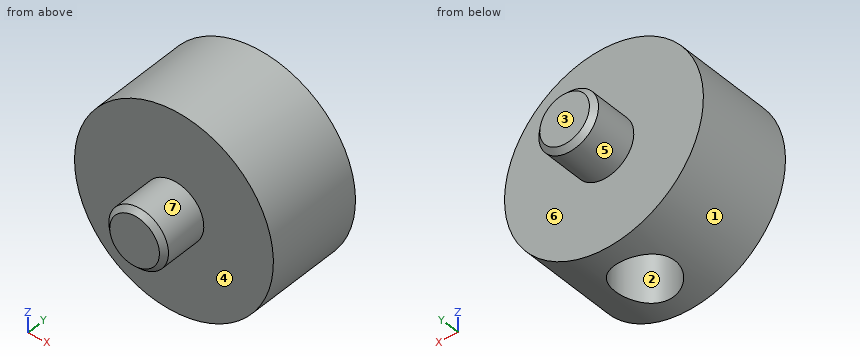
from build123d import *

# Parameters (mm, degrees)
SCHIZZO1_R                   = 10
ESTRUSIONE_ESTRUSIONE1_DEPTH = 10
ESTRUSIONE_ESTRUSIONE2_START = -14.8
SCHIZZO2_R                   = 3
ESTRUSIONE_ESTRUSIONE2_DEPTH = 19.6
TAGLIO_ESTRUSIONE1_START     = -0.5
SCHIZZO3_R                   = 3
TAGLIO_ESTRUSIONE1_DEPTH     = 9.5
SMUSSO1_SIZE                 = 0.5


with BuildPart() as part:
    # Schizzo1 → Estrusione-Estrusione1 (new body)
    with BuildSketch(Plane(origin=(0, 0, 0), x_dir=(1, 0, 0), z_dir=(0, 1, 0))):
        with Locations(Location((0, 0, 0), (0, 0, 270))):
            Circle(SCHIZZO1_R)
    extrude(amount=ESTRUSIONE_ESTRUSIONE1_DEPTH)

    # Schizzo2 → Estrusione-Estrusione2 (add)
    with BuildSketch(Plane.XZ.offset(ESTRUSIONE_ESTRUSIONE2_START)):
        with Locations(Location((0, 0, 0), (0, 0, 270))):
            Circle(SCHIZZO2_R)
    extrude(amount=ESTRUSIONE_ESTRUSIONE2_DEPTH)

    # Schizzo3 → Taglio-Estrusione1 (cut)
    with BuildSketch(Plane.XY.offset(TAGLIO_ESTRUSIONE1_START)):
        with Locations((0, 5)):
            Circle(SCHIZZO3_R)
    extrude(amount=-TAGLIO_ESTRUSIONE1_DEPTH, mode=Mode.SUBTRACT)

    # Smusso1
    smusso1_edges = [part.edges().sort_by_distance(p)[0] for p in [
        (0, -4.8, 3),
        (0, 14.8, 3),
    ]]
    chamfer(smusso1_edges, length=SMUSSO1_SIZE)


solid = part.part
Geometry check sheet. Reference: the model listing, model coordinates, mm. Face numbers are marked on the shaded views. A direction names the side the tool comes from. Round coordinates to 2 decimals unless told otherwise and drop trailing zeros. Loops run counter-clockwise (first coordinate to the right, second up) from the corner with the lowest first, then second, coordinate; pieces in that order, holes last. Notation, with made-up numbers: (68, 88) -> (118, 88) arc R15 ccw to (118, 104) -> close; hole circle Ø10 at (-19.75, -5.5). An arc over 180 degrees is marked (long way). Answer as a JSON object with one key per item and string values. Group by question number.
Item 1: Set-up check for the marked faces 1, 2, 3, 4 and 5: record each of +Z, -Z, +X, -X, +Y, -Y from which the full face is reachable in a straight line by a thin tool's end or side.
Item 2: Cross-section at C-C, the plane y = 10.5. Record the cut outline in (x, z), plus the area to 3 significant figures.
Item 3: Depth check by flat-ended pin: pin 1 Ø1 at (y, z) = (1.5, -2.5) entering from -X; pin 2 Ø3 at (y, z) = (9, -5) entering from +X; pin 3 Ø3 at (x, z) = (-4.5, 4.5) entering from -Y. Enter the tip coordinate at first touch or a pass-through.
Item 4: Cross-section at B-B, the plane x = 3.5. Record the cut outline in (y, z).
Item 5: Cross-section at A-A, the plane z = 0. Record the cut outline in (x, y).
Item 6: Release check for a two-part mould opening along Z. For the marked faces 6 and 7 record: pulls with the +Z half, pulls with the -Z half, needs draft (parallel to the pull), parting line crosses it, or undercut.
Item 7: Thickness scan on line 1 along Y through (x, z) = (0, -6); line 2 along Y through (x, z) = (-4.5, -8); line 3 along Z through (x, y) = (-0.25, 1). Record the ranges inside material, lowest first.
Item 8: Cross-section at D-D, the plane z = 8. Record the cut outline in (x, y).
Determined:
{
 "1": {"face 1": "+Y, -Y", "face 2": "-Z", "face 3": "+Z, -Z, +X, -X, +Y", "face 4": "-Y", "face 5": "+Y"},
 "2": {"outline": "circle Ø6 at (0, 0)", "area": "28.3 mm²"},
 "3": {"pin 1": "stops at x = -9.8", "pin 2": "stops at x = 9.37", "pin 3": "stops at y = 0"},
 "4": {"outline": "(0, -9.37) -> (10, -9.37) -> (10, 9.37) -> (0, 9.37) -> close"},
 "5": {"outline": "(-10, 0) -> (-3, 0) -> (-3, -4.3) -> (-2.5, -4.8) -> (2.5, -4.8) -> (3, -4.3) -> (3, 0) -> (10, 0) -> (10, 10) -> (3, 10) -> (3, 14.3) -> (2.5, 14.8) -> (-2.5, 14.8) -> (-3, 14.3) -> (-3, 10) -> (-10, 10) -> close"},
 "6": {"face 6": "needs draft", "face 7": "parting line crosses it"},
 "7": {"line 1": "y = 0 to 2, 8 to 10", "line 2": "y = 0 to 10", "line 3": "z = -10 to 10"},
 "8": {"outline": "(-6, 0) -> (6, 0) -> (6, 10) -> (-6, 10) -> close"}
}
